Autodesk Inventor part; units mm, degrees
ref_plane "YZ Plane" through (0, 0, 0) normal (1, 0, 0) x (0, 1, 0)
ref_plane "XZ Plane" through (0, 0, 0) normal (0, 1, 0) x (-1, 0, 0)
ref_plane "XY Plane" through (0, 0, 0) normal (0, 0, 1) x (1, 0, 0)
sketch "Esquisse1" plane through (0, 0, 0) normal (1, 0, 0) x (0, 1, 0)
  line L0 (0, 0) -> (25, 0)
  line L1 (25, 0) -> (25, -30)
  line L2 (25, -30) -> (0, -30)
  line L3 (0, -30) -> (0, 0)
  dimension "d0" = 25
  dimension "d1" = 30
extrude "Extrusion1" add sketch "Esquisse1" along normal blind 243
sketch "Esquisse2" plane through (0, 25, 0) normal (0, 1, 0) x (1, 0, 0)
  circle A0 centre (15, 15) radius 1.5
  line L0 (0, 30) -> (0, 0)
  circle A1 centre (234, 15) radius 1.5
  dimension "d4" = 3
  dimension "d5" = 15
  dimension "d6" = 3
  dimension "d7" = 219
extrude "Extrusion2" cut sketch "Esquisse2" against normal blind 25 from surface at 0
sketch "Esquisse3" plane through (0, 0, 0) normal (0, 0, 1) x (1, 0, 0)
  line L0 (0, 25) -> (243, 25)
  line L1 (0, 25) -> (40, 25)
  line L2 (40, 25) -> (40, 12.5)
  line L3 (40, 12.5) -> (0, 12.5)
  line L4 (0, 12.5) -> (0, 25)
  line L5 (243, 25) -> (203, 25)
  line L6 (203, 25) -> (203, 12.5)
  line L7 (203, 12.5) -> (243, 12.5)
  line L8 (243, 12.5) -> (243, 25)
  point P0 (0, 0)
  dimension "d10" = 12.5
  dimension "d11" = 40
  dimension "d12" = 40
extrude "Extrusion3" cut sketch "Esquisse3" against normal through all
properties part number "Bras_avant"
Geometry: final body of the model. Coordinates: model frame, mm. A direction names the side the tool comes from. Round coordinates to 2 decimals unless told otherwise and drop trailing zeros. Order: outer loops, then holes, each group sorted by start corner. A loop starts at its lowest first (then second) coordinate and runs counter-clockwise, first axis right, second up. Notation, with made-up numbers: (56.5, 22.25) -> (104.5, 22.25) arc R11 ccw to (104.5, 31.25) -> close; hole circle Ø3 at (21.5, 31). An arc over 180 degrees is marked (long way). Use one line per item in the form item = value. Start each with the question number.
1. Reachability of faces 1 (the face through (40, 19, -15)), 2 (the face through (203, 19, -15)), 3 (the face through (120, 25, -15)) from +Z, -Z, +X, -X, +Y, -Y: full face, straight path, thin tool, end or side. Return the list, or none.
2. Line query: probe 1 along X at (y, z) = (9, -15); probe 2 along Z at (x, y) = (15, 3.5); probe 3 along X at (y, z) = (21, -26.75). Output: solid intervals per line, ascending.
3. Pin query (flat end, axial travel): pin 1 Ø9 at (x, z) = (17, -9.5) entering from +Y; pin 2 Ø10 at (y, z) = (20, -12) entering from +X; pin 3 Ø6 at (y, z) = (16.5, -19) entering from -X. Return the tip coordinate at first contact, or that it passes through.
4. Cut plane A-A (z = -10.5). Return the cut outline in (x, y).
5. Cut plane C-C (y = 17.75). Return the cut outline in (x, z), then the cut area to 3 significant figures.
6. Cut plane B-B (x = 21.5). Return the cut outline in (y, z).
Solution:
q1.face_1 = +Z, -Z, -X, +Y
q1.face_2 = +Z, -Z, +X, +Y
q1.face_3 = +Z, -Z, +X, -X, +Y
q2.probe_1 = 0 to 13.5, 16.5 to 232.5, 235.5 to 243
q2.probe_2 = -30 to -16.5, -13.5 to 0
q2.probe_3 = 40 to 203
q3.pin_1 = 12.5
q3.pin_2 = 203
q3.pin_3 = 40
q4.outline = (0, 0) -> (243, 0) -> (243, 12.5) -> (203, 12.5) -> (203, 25) -> (40, 25) -> (40, 12.5) -> (0, 12.5) -> close
q5.outline = (40, -30) -> (203, -30) -> (203, 0) -> (40, 0) -> close
q5.area = 4,890 mm^2
q6.outline = (0, -30) -> (12.5, -30) -> (12.5, 0) -> (0, 0) -> close
